Check sheet for the modelled part. Datum: model origin and axes. Units: mm. Face numbers are marked on the shaded views. A direction names the side the tool comes from. Round coordinates to 2 decimals unless told otherwise and drop trailing zeros. Order: outer loops, then holes, each group sorted by start corner. A loop starts at its lowest first (then second) coordinate and runs counter-clockwise, first axis right, second up. Notation, with made-up numbers: (45.5, -36) -> (99.5, -36) arc R11 ccw to (99.5, -28) -> close; hole circle Ø1 at (-29, 49). An arc over 180 degrees is marked (long way). Answer in a Markdown table with one row per item.
from build123d import *

# Parameters (mm, degrees)
F0_W        = 50.8
F0_H        = 114.3
F1_DEPTH    = 15.748
F2_W        = 9.652
F2_H        = 12.7
F3_DEPTH    = 25.4
F4_R        = 12.7
F5_T1_DEPTH = 15.748
F7_DEPTH    = 15.748
F8_R        = 15.875
F9_DEPTH    = 3.048
F10_R       = 7.9375
F11_DEPTH   = 25.4


# Not quite as in the source:
# - a fillet or chamfer that OpenCascade refuses, or shapes differently, is made with other operations: its cross-section is extruded or revolved along the edge and cut away or added


with BuildPart() as f1:
    # F0 (on Top) → F1 (new body)
    with BuildSketch(Plane.XY):
        with Locations((-2.3709591478, 9.3886919219)):
            Rectangle(F0_W, F0_H)
    extrude(amount=F1_DEPTH)

    # F2 (on face) → F3 (cut)
    with BuildSketch(Plane.XY.offset(15.748)):
        with Locations((-2.3709591478, -41.4113080781)):
            Rectangle(F2_W, F2_H)
        with Locations((-2.3709591478, 60.1886919219)):
            Rectangle(F2_W, F2_H)
    extrude(amount=-F3_DEPTH, mode=Mode.SUBTRACT)

    # F4
    f4_edges = [f1.edges().sort_by_distance(p)[0] for p in [
        (-27.770959, 66.538692, 7.874),
        (23.029041, 66.538692, 7.874),
        (-27.770959, -47.761308, 7.874),
        (23.029041, -47.761308, 7.874),
    ]]
    fillet(f4_edges, radius=F4_R)

    # F5: fillet of radius 5.08 on 4 edges, made by hand

    # F5_s2 → F5_t1 (join)
    with BuildSketch(Plane.XY):
        with BuildLine():
            ThreePointArc((-2.6249591478, 53.8386919219), (0.9671433006, 55.3265894735), (2.4550408522, 58.9186919219))
            Line((2.4550408522, 58.9186919219), (2.4550408522, 53.8386919219))
            Line((2.4550408522, 53.8386919219), (-2.6249591478, 53.8386919219))
        make_face()
        with BuildLine():
            ThreePointArc((-7.1969591478, 58.9186919219), (-5.7090615962, 55.3265894735), (-2.1169591478, 53.8386919219))
            Line((-2.1169591478, 53.8386919219), (-7.1969591478, 53.8386919219))
            Line((-7.1969591478, 53.8386919219), (-7.1969591478, 58.9186919219))
        make_face()
        with BuildLine():
            ThreePointArc((-2.6249591478, -35.0613080781), (0.9671433006, -36.5492056297), (2.4550408522, -40.1413080781))
            Line((2.4550408522, -40.1413080781), (2.4550408522, -35.0613080781))
            Line((2.4550408522, -35.0613080781), (-2.6249591478, -35.0613080781))
        make_face()
        with BuildLine():
            ThreePointArc((-7.1969591478, -40.1413080781), (-5.7090615962, -36.5492056297), (-2.1169591478, -35.0613080781))
            Line((-2.1169591478, -35.0613080781), (-7.1969591478, -35.0613080781))
            Line((-7.1969591478, -35.0613080781), (-7.1969591478, -40.1413080781))
        make_face()
    extrude(amount=F5_T1_DEPTH)

    # F6 (on face) → F7 (join)
    with BuildSketch(Plane.YZ.offset(23.0290408522)):
        with BuildLine():
            Line((34.7886919219, 15.748), (34.7886919219, 34.798))
            ThreePointArc((34.7886919219, 34.798), (9.3886919219, 60.198), (-16.0113080781, 34.798))
            Line((-16.0113080781, 34.798), (-16.0113080781, 15.748))
            Line((-16.0113080781, 15.748), (34.7886919219, 15.748))
        make_face()
    extrude(amount=-F7_DEPTH)

    # F8 (on face) → F9 (cut)
    with BuildSketch(Plane.YZ.offset(23.0290408522)):
        with Locations((9.3886919219, 34.798)):
            Circle(F8_R)
    extrude(amount=-F9_DEPTH, mode=Mode.SUBTRACT)

    # F10 (on face) → F11 (cut)
    with BuildSketch(Plane.YZ.offset(19.9810408522)):
        with Locations((9.3886919219, 34.798)):
            Circle(F10_R)
    extrude(amount=-F11_DEPTH, mode=Mode.SUBTRACT)


solid = f1.part
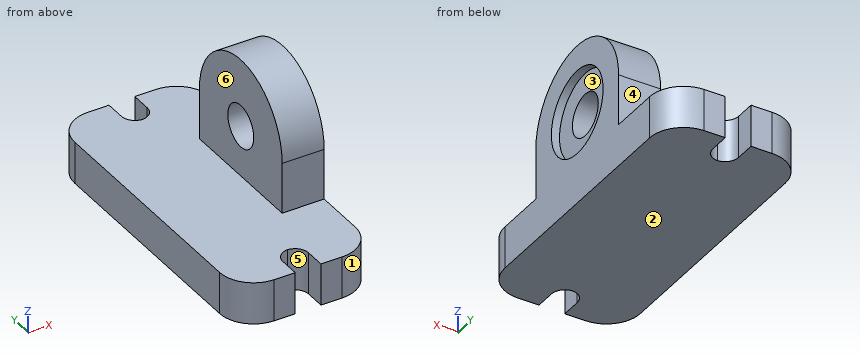
Item 1: Cross-section at C-C (y = 5). Record the boundary of the cut face in (x, z).
Result sheet:
| item | result |
|---|---|
| outline | (-27.77, 0) -> (23.03, 0) -> (23.03, 19.54) -> (19.98, 19.54) -> (19.98, 28.18) -> (7.28, 28.18) -> (7.28, 15.75) -> (-27.77, 15.75) -> close; (7.28, 41.41) -> (19.98, 41.41) -> (19.98, 50.05) -> (23.03, 50.05) -> (23.03, 59.82) -> (7.28, 59.82) -> close |
Item 2: Depth check by flat-ended pin: P1, Ø4.5, axis at x = 17, z = 29, coming from the -Y side; P2, Ø4, axis at y = 62.5, z = 4.5, coming from the +X side; P3, Ø6, axis at y = 63.5, z = 10, coming from the -X side; P4, Ø3, axis at x = -3.5, y = 11, coming from the -Z side. Enter the tip coordinate at first touch or a pass-through.
Result sheet:
| item | result |
|---|---|
| P1 | stops at y = -16.01 |
| P2 | stops at x = 21.14 |
| P3 | stops at x = -25.88 |
| P4 | stops at z = 0 |
Item 3: Cross-section at D-D (x = -9). Record the boundary of the cut face in (y, z).
Result sheet:
| item | result |
|---|---|
| outline | (-47.76, 0) -> (66.54, 0) -> (66.54, 15.75) -> (-47.76, 15.75) -> close |
Item 4: Set-up check for the marked faces 4, 5 and 6: record each of +Z, -Z, +X, -X, +Y, -Y from which the full face is reachable in a straight line by a thin tool's end or side.
Result sheet:
| item | result |
|---|---|
| face 4 | +Z, +X, -X, +Y |
| face 5 | +Z, -Z, -Y |
| face 6 | +Z, -X, +Y, -Y |
Item 5: Scan lines: line 1 (Z direction, x = -8.5, y = 47.5); line 2 (X direction, y = 16.5, z = 44.5); line 3 (X direction, y = 19, z = 51). Record each from-to range of solid material in increasing order. Write a range as [from, to].
Result sheet:
| item | result |
|---|---|
| line 1 | z = [0, 15.75] |
| line 2 | x = [7.28, 19.98] |
| line 3 | x = [7.28, 23.03] |
Item 6: Cross-section at A-A (x = 9). Record the boundary of the cut face in (y, z) (1 decimal), and give its area (3 significant figures).
Result sheet:
| item | result |
|---|---|
| outline | (-47.8, 0) -> (66.5, 0) -> (66.5, 15.7) -> (34.8, 15.7) -> (34.8, 34.8) arc R25.4 ccw to (-16, 34.8) -> (-16, 15.7) -> (-47.8, 15.7) -> close; hole circle Ø15.9 at (9.4, 34.8) |
| area | 3,580 mm^2 |
Item 7: Cross-section at B-B (z = 13). Record the boundary of the cut face in (x, y), and give its area (3 significant figures).
Result sheet:
| item | result |
|---|---|
| outline | (-27.77, -35.06) arc R12.7 ccw to (-15.07, -47.76) -> (-7.2, -47.76) -> (-7.2, -40.14) arc R5.08 cw to (-2.37, -35.07) arc R5.08 cw to (2.46, -40.14) -> (2.46, -47.76) -> (10.33, -47.76) arc R12.7 ccw to (23.03, -35.06) -> (23.03, 53.84) arc R12.7 ccw to (10.33, 66.54) -> (2.46, 66.54) -> (2.46, 58.92) arc R5.08 cw to (-2.37, 53.85) arc R5.08 cw to (-7.2, 58.92) -> (-7.2, 66.54) -> (-15.07, 66.54) arc R12.7 ccw to (-27.77, 53.84) -> close |
| area | 5,440 mm^2 |
Item 8: Mould release check, pull along Y, two halves, no side actions. Record for the marked faces 1, 2 and 3: pulls with the +Y half, pulls with the -Y half, needs draft (parallel to the pull), parting line crosses it, or undercut.
Result sheet:
| item | result |
|---|---|
| face 1 | pulls with the -Y half |
| face 2 | needs draft |
| face 3 | undercut |
